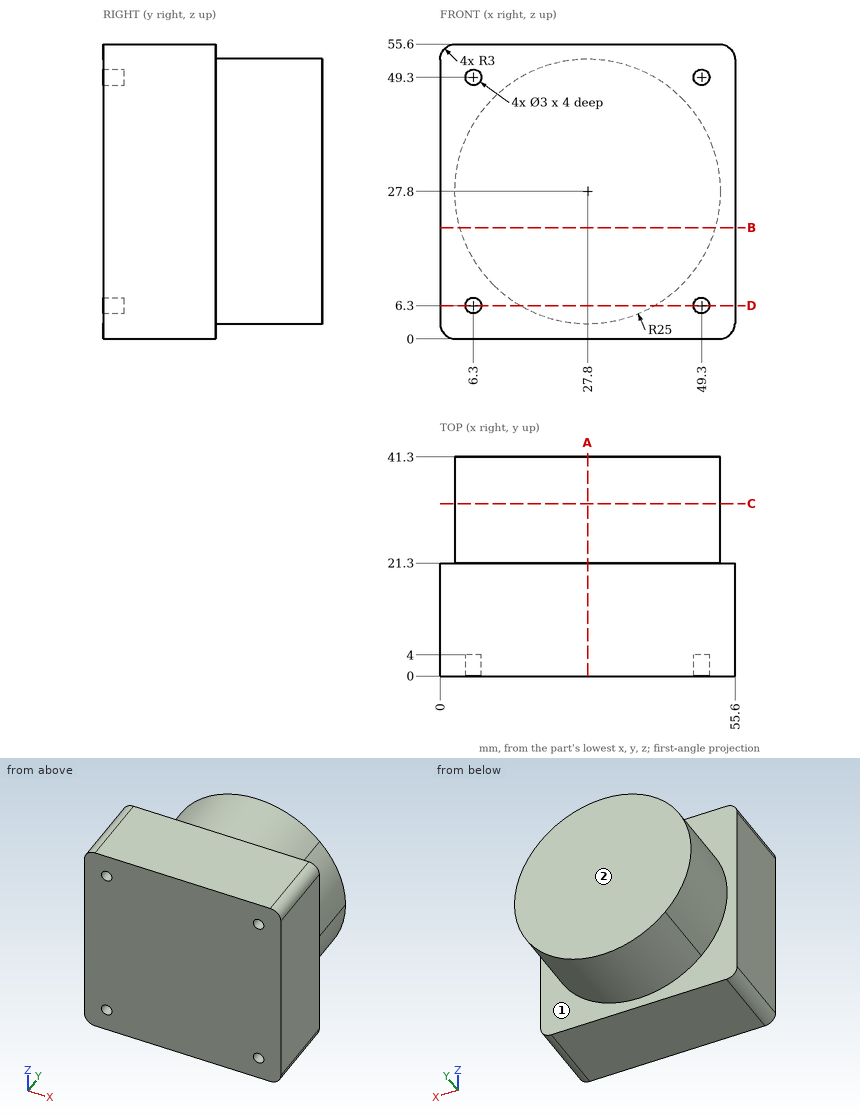
Geometry check sheet. Reference: drawing and pictorial views, mm from the part's lowest x, y, z. A direction names the side the tool comes from. Round coordinates to 2 decimals unless told otherwise and drop trailing zeros. Loops run counter-clockwise (first coordinate to the right, second up) from the corner with the lowest first, then second, coordinate; pieces in that order, holes last. Notation, with made-up numbers: (29.25, 36.5) - (75.25, 36.5) arc R15 cw to (75.25, 40.5) - close; hole circle Ø8 at (52.5, 23). An arc over 180 degrees is marked (long way). Answer as CSV lines item,"result".
(1) Depth check by flat-ended pin: pin 1 Ø1 at (y, z) = (19.5, 15.5) entering from -X; pin 2 Ø6 at (y, z) = (28.5, 38) entering from -X; pin 3 Ø0.9 at (x, z) = (49, 5.5) entering from -Y; pin 4 Ø4 at (x, z) = (6.3, 49.3) entering from +Y. Enter the tip coordinate at first touch or a pass-through.
Output values:
pin 1,"stops at x = 0"
pin 2,"stops at x = 3.86"
pin 3,"stops at y = 4"
pin 4,"stops at y = 21.3"
(2) Cross-section at D-D, the plane z = 6.3. Enter the section's corners in (x, y).
Output values:
outline,"(0, 0) - (4.8, 0) - (4.8, 4) - (7.8, 4) - (7.8, 0) - (47.8, 0) - (47.8, 4) - (50.8, 4) - (50.8, 0) - (55.6, 0) - (55.6, 21.3) - (40.56, 21.3) - (40.56, 41.3) - (15.04, 41.3) - (15.04, 21.3) - (0, 21.3) - close"
(3) Material ranges on line 1 along Z through (x, y) = (49.3, 2.6); line 2 along X through (y, z) = (1, 49); line 3 along X through (y, z) = (31.5, 28.5), recorded low to high.
Output values:
line 1,"z = 0 to 4.8, 7.8 to 47.8, 50.8 to 55.6"
line 2,"x = 0 to 4.83, 7.77 to 47.83, 50.77 to 55.6"
line 3,"x = 2.81 to 52.79"
(4) Cross-section at A-A, the plane x = 27.8. Enter the section's corners in (y, z), and give its area (3 significant figures).
Output values:
outline,"(0, 0) - (21.3, 0) - (21.3, 2.8) - (41.3, 2.8) - (41.3, 52.8) - (21.3, 52.8) - (21.3, 55.6) - (0, 55.6) - close"
area,"2,180 mm²"
(5) Cross-section at B-B, the plane z = 21. Enter the section's corners in (x, y), and give its area (3 significant figures).
Output values:
outline,"(0, 0) - (55.6, 0) - (55.6, 21.3) - (51.86, 21.3) - (51.86, 41.3) - (3.74, 41.3) - (3.74, 21.3) - (0, 21.3) - close"
area,"2,150 mm²"
(6) Cross-section at C-C, the plane y = 32.5. Enter the section's corners in (x, z), and give its area (3 significant figures).
Output values:
outline,"circle Ø50 at (27.8, 27.8)"
area,"1,960 mm²"
(7) Set-up check for the marked faces 1 and 2: record each of +Z, -Z, +X, -X, +Y, -Y from which the full face is reachable in a straight line by a thin tool's end or side.
Output values:
face 1,"+Y"
face 2,"+Z, -Z, +X, -X, +Y"
